from build123d import *

# Parameters (mm, degrees)
ESQUISSE1_W             = 90
ESQUISSE1_H             = 65
ESQUISSE1_R             = 7
ESQUISSE1_R_2           = 13
BOSS_EXTRU_1_DEPTH      = 8
BOSS_EXTRU_2_START      = -8
ESQUISSE2_R             = 13
BOSS_EXTRU_2_DEPTH      = 3
ESQUISSE3_R             = 7
ESQUISSE3_R_2           = 1.5
ENL_V_MAT_EXTRU_1_DEPTH = 4
ENL_V_START             = -8
ESQUISSE4_R             = 8
ENL_V_MAT_EXTRU_2_DEPTH = 5
ESQUISSE5_W             = 45
ESQUISSE5_H             = 8
ENL_V_MAT_EXTRU_3_DEPTH = 9
ESQUISSE6_R             = 1.65
ENL_V_MAT_EXTRU_4_DEPTH = 10
ESQUISSE7_R             = 1.65
ENL_V_MAT_EXTRU_5_DEPTH = 10


with BuildPart() as part:
    # Esquisse1 → Boss.-Extru.1 (new body)
    with BuildSketch(Plane.XY):
        with Locations((45, 32.5)):
            Rectangle(ESQUISSE1_W, ESQUISSE1_H)
        with Locations((70, 20)):
            Circle(ESQUISSE1_R, mode=Mode.SUBTRACT)
        with Locations((17, 20)):
            Circle(ESQUISSE1_R_2, mode=Mode.SUBTRACT)
        with Locations((25, 48)):
            Circle(ESQUISSE1_R_2, mode=Mode.SUBTRACT)
    extrude(amount=BOSS_EXTRU_1_DEPTH)

    # Esquisse2 → Boss.-Extru.2 (add)
    with BuildSketch(Plane(origin=(0, 0, 0), x_dir=(-1, 0, 0), z_dir=(0, 0, -1)).offset(BOSS_EXTRU_2_START)):
        with Locations((-25, 48)):
            Circle(ESQUISSE2_R)
    extrude(amount=BOSS_EXTRU_2_DEPTH)

    # Esquisse3 → Enlèv. mat.-Extru.1 (cut, through all)
    with BuildSketch(Plane(origin=(0, 0, 5), x_dir=(-1, 0, 0), z_dir=(0, 0, -1))):
        with Locations((-25, 48)):
            Circle(ESQUISSE3_R)
        with Locations((-15, 48)):
            Circle(ESQUISSE3_R_2)
        with Locations((-25, 38)):
            Circle(ESQUISSE3_R_2)
        with Locations((-35, 48)):
            Circle(ESQUISSE3_R_2)
        with Locations((-25, 58)):
            Circle(ESQUISSE3_R_2)
    extrude(amount=-ENL_V_MAT_EXTRU_1_DEPTH, mode=Mode.SUBTRACT)

    # Esquisse4 → Enlèv. mat.-Extru.2 (cut)
    with BuildSketch(Plane.XY.offset(8).offset(ENL_V_START)):
        with Locations((70, 20)):
            Circle(ESQUISSE4_R)
    extrude(amount=ENL_V_MAT_EXTRU_2_DEPTH, mode=Mode.SUBTRACT)

    # Esquisse5 → Enlèv. mat.-Extru.3 (cut, through all)
    with BuildSketch(Plane(origin=(0, 0, 0), x_dir=(-1, 0, 0), z_dir=(0, 0, -1))):
        with Locations((-67.5, 61)):
            Rectangle(ESQUISSE5_W, ESQUISSE5_H)
    extrude(amount=-ENL_V_MAT_EXTRU_3_DEPTH, mode=Mode.SUBTRACT)

    # Esquisse6 → Enlèv. mat.-Extru.4 (cut)
    with BuildSketch(Plane.ZY):
        with Locations((4, 45)):
            Circle(ESQUISSE6_R)
        with Locations((4, 7)):
            Circle(ESQUISSE6_R)
    extrude(amount=-ENL_V_MAT_EXTRU_4_DEPTH, mode=Mode.SUBTRACT)

    # Esquisse7 → Enlèv. mat.-Extru.5 (cut)
    with BuildSketch(Plane(origin=(0, 57, 0), x_dir=(1, 0, 0), z_dir=(0, 1, 0))):
        with Locations((85, -4)):
            Circle(ESQUISSE7_R)
        with Locations((55, -4)):
            Circle(ESQUISSE7_R)
    extrude(amount=-ENL_V_MAT_EXTRU_5_DEPTH, mode=Mode.SUBTRACT)


solid = part.part
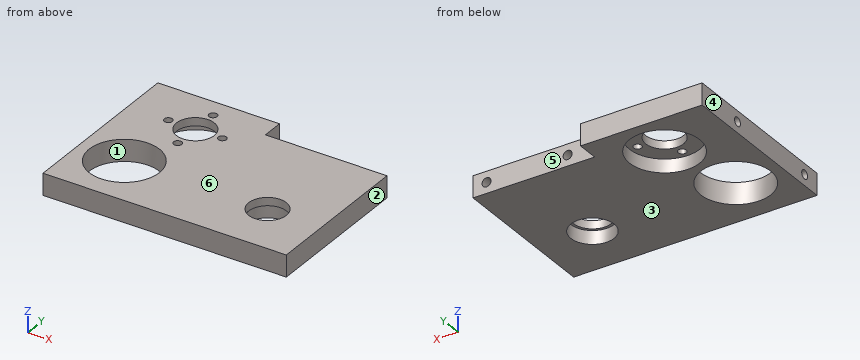
Work out the finished part from the listing and answer in its coordinate system (mm). Face numbers are marked on the shaded views. A direction names the side the tool comes from. Round coordinates to 2 decimals unless told otherwise and drop trailing zeros. Write each loop counter-clockwise with the first axis right and the second up, starting at its lowest first coordinate (ties: lowest second). Pieces come first, ordered by that corner, then holes. Notation, with made-up numbers: M 51.25,28.25 L 82.25,28.25 A9 cw 82.25,33.25 Z; hole C -16,-34.75 d5. An arc over 180 degrees is marked long. Use a Markdown table: item, result.
1) Consider line 1 (Y direction, x = 70, z = 6.7); line 2 (Z direction, x = 55, y = 53.5); line 3 (Y direction, x = 25, z = 7.1). Determine where each line is inside the solid, lowest interval first. Write a range as [from, to].
Taken from the geometry:
| item | result |
|---|---|
| line 1 | y = [0, 13], [27, 57] |
| line 2 | z = [0, 2.35], [5.65, 8] |
| line 3 | y = [0, 9.75], [30.25, 36.5], [39.5, 41], [55, 56.5], [59.5, 65] |
2) Which of the six approach directions +Z, -Z, +X, -X, +Y, -Y give full straight-line access (tool end or side, diameter ignored) to the marked faces 5 and 6?
Taken from the geometry:
| item | result |
|---|---|
| face 5 | +Z, -Z, +X, +Y |
| face 6 | +Z, +X, -X, +Y, -Y |
3) The part is cut by section A-A on z = 6.75. Give the vertices of the cut face in (x, y).
Taken from the geometry:
| item | result |
|---|---|
| outline | M 0,0 L 90,0 L 90,57 L 45,57 L 45,65 L 0,65 Z; hole C 17,20 d26; hole C 15,48 d3; hole C 25,48 d14; hole C 25,38 d3; hole C 25,58 d3; hole C 35,48 d3; hole C 70,20 d14 |
4) Flat-ended cylindrical pins translate along their axes: pin 1 (11 mm diameter, centred on x = 25, y = 48, fed in from +Z); pin 2 (3.5 mm diameter, centred on y = 44.5, z = 4.5, fed in from -X); pin 3 (3.5 mm diameter, centred on x = 55.5, z = 3.5, fed in from +Y); pin 4 (2.5 mm diameter, centred on y = 62.5, z = 5.5, fed in from +X). Find the tip coordinate at first contact, or state that the pin passes through.
Taken from the geometry:
| item | result |
|---|---|
| pin 1 | passes through |
| pin 2 | stops at x = 0 |
| pin 3 | stops at y = 57 |
| pin 4 | stops at x = 45 |
5) Determine the mould class of the marked faces 1, 2, 3 and 4 for opening direction X: pulls with the +X half, pulls with the -X half, needs draft (parallel to the pull), parting line crosses it, or undercut.
Taken from the geometry:
| item | result |
|---|---|
| face 1 | undercut |
| face 2 | pulls with the +X half |
| face 3 | needs draft |
| face 4 | pulls with the -X half |
6) The part is cut by section D-D on x = 9. Give the vertices of the cut face in (y, z).
Taken from the geometry:
| item | result |
|---|---|
| outline | M 0,0 L 9.75,0 L 9.75,8 L 0,8 Z; M 30.25,0 L 65,0 L 65,8 L 30.25,8 Z; hole C 7,4 d3.3; hole C 45,4 d3.3 |
7) The part is cut by section B-B on x = 70. Give the vertices of the cut face in (y, z), plus the area to 3 significant figures.
Taken from the geometry:
| item | result |
|---|---|
| outline | M 0,0 L 12,0 L 12,5 L 13,5 L 13,8 L 0,8 Z; M 27,5 L 28,5 L 28,0 L 57,0 L 57,8 L 27,8 Z |
| area | 334 mm2 |
8) The part is cut by section C-C on y = 20. Give the vertices of the cut face in (x, z), plus the area to 3 significant figures.
Taken from the geometry:
| item | result |
|---|---|
| outline | M 0,0 L 4,0 L 4,8 L 0,8 Z; M 30,0 L 62,0 L 62,5 L 63,5 L 63,8 L 30,8 Z; M 77,5 L 78,5 L 78,0 L 90,0 L 90,8 L 77,8 Z |
| area | 390 mm2 |
